The listing builds one solid part. Answer for the finished solid, in the listing's coordinates (mm). A direction names the side the tool comes from. Give positions to 0.01 mm unless a question says otherwise; leave off trailing zeros. Order: outer loops, then holes, each group sorted by start corner. A loop starts at its lowest first (then second) coordinate and runs counter-clockwise, first axis right, second up. Notation, with made-up numbers: (86, 67.25) - (136, 67.25) arc R11 ccw to (136, 79.25) - close; hole circle Ø7 at (4, 67). An arc over 180 degrees is marked (long way). Use a Markdown table: item, result. Add a question column.
1) Flat-ended cylindrical pins translate along their axes: pin 1 (2.5 mm diameter, centred on x = 62, y = 129, fed in from -Z); pin 2 (4 mm diameter, centred on x = 17, y = 22, fed in from +Z); pin 3 (5 mm diameter, centred on x = 61, y = 9, fed in from +Z); pin 4 (2 mm diameter, centred on x = 61, y = 9, fed in from +Z). Find the tip coordinate at first contact, or state that the pin passes through.
2) Find section C-C, the plane y = 83.5. Determine the outline of the cut face in (x, z), plus the area to 3 significant figures.
3) The mould has two halves that part along X. Classify faces 4 (the face through (1, 80, 70)), 5 (the face through (0, 67, 35)), 6 (the face through (58.85, 131.373, 33.031)), 7 (the face through (9.521, 131.966, 33.031)): released by +X, released by -X, zero draft, split by the parting line, or undercut.
4) For faces 1 (the face through (57.185, 10.201, 33.031)), 2 (the face through (60, 168, 2)), 3 (the face through (68, 79, 36)), determine the directions among +Z, -Z, +X, -X, +Y, -Y from which every point of the face is accessible in a straight line to the end or side of a thin tool.
5) Find section A-A, the plane z = 52.5. State how many separate pieces and enclosed holes the cut face has, plus the area to 3 significant figures.
6) Straight lines are drawn through the part: line 1 (Y direction, x = 61, z = 67.85); line 2 (Y direction, x = 61, z = 43); line 3 (X direction, y = 128, z = 67.5). For each, find the intervals that lie inside material, in ascending order.
7) Find section B-B, the plane y = 145. Determine the outline of the cut face in (x, z), plus the area to 3 significant figures.
from build123d import *

# Parameters (mm, degrees)
CROQUIS1_W              = 70
CROQUIS1_H              = 160
SALIENTE_EXTRUIR1_DEPTH = 70
VACIADO1_T              = -2
CROQUIS2_W              = 13
CROQUIS2_H              = 19
CORTAR_EXTRUIR1_DEPTH   = 188.413980268
CORTAR_EXTRUIR2_DEPTH   = 188.413980268
CORTAR_EXTRUIR3_DEPTH   = 188.413980268
CROQUIS5_R              = 5
CROQUIS5_R_2            = 3
SALIENTE_EXTRUIR2_DEPTH = 67
CROQUIS6_R              = 3.05
CROQUIS6_R_2            = 1.4
SALIENTE_EXTRUIR3_DEPTH = 2
SALIENTE_EXTRUIR4_DEPTH = 4
CROQUIS8_R              = 4
CORTAR_EXTRUIR4_DEPTH   = 67


with BuildPart() as part:
    # Croquis1 → Saliente-Extruir1 (new body)
    with BuildSketch(Plane.XY):
        with Locations((35, 80)):
            Rectangle(CROQUIS1_W, CROQUIS1_H)
    extrude(amount=SALIENTE_EXTRUIR1_DEPTH)

    # Vaciado1
    vaciado1_openings = [part.faces().sort_by_distance(p)[0] for p in [
        (35, 80, 70),
    ]]
    offset(amount=VACIADO1_T, openings=vaciado1_openings, kind=Kind.INTERSECTION)

    # Croquis2 → Cortar-Extruir1 (cut, through all)
    with BuildSketch(Plane.XY.offset(2)):
        with Locations((60, 147)):
            Rectangle(CROQUIS2_W, CROQUIS2_H)
    extrude(amount=-CORTAR_EXTRUIR1_DEPTH, mode=Mode.SUBTRACT)

    # Croquis3 → Cortar-Extruir2 (cut, through all)
    with BuildSketch(Plane.XY.offset(2)):
        with BuildLine():
            Line((29.75, 14.573472877), (40.25, 14.573472877))
            ThreePointArc((40.25, 14.573472877), (44, 10.823472877), (40.25, 7.073472877))
            Line((40.25, 7.073472877), (29.75, 7.073472877))
            ThreePointArc((29.75, 7.073472877), (26, 10.823472877), (29.75, 14.573472877))
        make_face()
    extrude(amount=-CORTAR_EXTRUIR2_DEPTH, mode=Mode.SUBTRACT)

    # Croquis4 → Cortar-Extruir3 (cut, through all)
    with BuildSketch(Plane(origin=(2, 0, 0), x_dir=(0, 0, -1), z_dir=(1, 0, 0))):
        with BuildLine():
            Line((-28, 148), (-20, 148))
            ThreePointArc((-20, 148), (-17, 145), (-20, 142))
            Line((-20, 142), (-28, 142))
            ThreePointArc((-28, 142), (-31, 145), (-28, 148))
        make_face()
    extrude(amount=-CORTAR_EXTRUIR3_DEPTH, mode=Mode.SUBTRACT)

    # Croquis5 → Saliente-Extruir2 (add)
    # profile 1 of 4: a face of its own
    with BuildSketch(Plane.XY.offset(2)):
        with Locations(Location((9, 128, 0), (0, 0, 180))):
            Circle(CROQUIS5_R)
        with Locations((9, 128)):
            Circle(CROQUIS5_R_2, mode=Mode.SUBTRACT)
    # profile 2 of 4: a face of its own
    with BuildSketch(Plane.XY.offset(2)):
        with Locations(Location((9, 9, 0), (0, 0, 180))):
            Circle(CROQUIS5_R)
        with Locations((9, 9)):
            Circle(CROQUIS5_R_2, mode=Mode.SUBTRACT)
    # profile 3 of 4: a face of its own
    with BuildSketch(Plane.XY.offset(2)):
        with Locations(Location((61, 128, 0), (0, 0, 180))):
            Circle(CROQUIS5_R)
        with Locations((61, 128)):
            Circle(CROQUIS5_R_2, mode=Mode.SUBTRACT)
    # profile 4 of 4: a face of its own
    with BuildSketch(Plane.XY.offset(2)):
        with Locations(Location((61, 9, 0), (0, 0, 180))):
            Circle(CROQUIS5_R)
        with Locations((61, 9)):
            Circle(CROQUIS5_R_2, mode=Mode.SUBTRACT)
    extrude(amount=SALIENTE_EXTRUIR2_DEPTH)

    # Croquis6 → Saliente-Extruir3 (add)
    # profile 1 of 4: a face of its own
    with BuildSketch(Plane.XY.offset(69)):
        with Locations((9, 128)):
            Circle(CROQUIS6_R)
        with Locations((9, 128)):
            Circle(CROQUIS6_R_2, mode=Mode.SUBTRACT)
    # profile 2 of 4: a face of its own
    with BuildSketch(Plane.XY.offset(69)):
        with Locations((61, 128)):
            Circle(CROQUIS6_R)
        with Locations((61, 128)):
            Circle(CROQUIS6_R_2, mode=Mode.SUBTRACT)
    # profile 3 of 4: a face of its own
    with BuildSketch(Plane.XY.offset(69)):
        with Locations((61, 9)):
            Circle(CROQUIS6_R)
        with Locations((61, 9)):
            Circle(CROQUIS6_R_2, mode=Mode.SUBTRACT)
    # profile 4 of 4: a face of its own
    with BuildSketch(Plane.XY.offset(69)):
        with Locations((9, 9)):
            Circle(CROQUIS6_R)
        with Locations((9, 9)):
            Circle(CROQUIS6_R_2, mode=Mode.SUBTRACT)
    extrude(amount=-SALIENTE_EXTRUIR3_DEPTH)

    # Croquis7 → Saliente-Extruir4 (add)
    # profile 1 of 2: a face of its own
    with BuildSketch(Plane(origin=(0, 0, 0), x_dir=(-1, 0, 0), z_dir=(0, 0, -1))):
        with BuildLine():
            Line((-70, 160), (-60, 160))
            Line((-60, 160), (-60, 176))
            ThreePointArc((-60, 176), (-61.171572875, 178.828427125), (-64, 180))
            Line((-64, 180), (-66, 180))
            ThreePointArc((-66, 180), (-68.828427125, 178.828427125), (-70, 176))
            Line((-70, 176), (-70, 160))
        make_face()
        with BuildLine():
            Line((-66, 177.5), (-64, 177.5))
            ThreePointArc((-64, 177.5), (-62.5, 176), (-64, 174.5))
            Line((-64, 174.5), (-66, 174.5))
            ThreePointArc((-66, 174.5), (-67.5, 176), (-66, 177.5))
        make_face(mode=Mode.SUBTRACT)
    # profile 2 of 2: a face of its own
    with BuildSketch(Plane(origin=(0, 0, 0), x_dir=(-1, 0, 0), z_dir=(0, 0, -1))):
        with BuildLine():
            Line((0, 160), (-10, 160))
            Line((-10, 160), (-10, 176))
            ThreePointArc((-10, 176), (-8.828427125, 178.828427125), (-6, 180))
            Line((-6, 180), (-4, 180))
            ThreePointArc((-4, 180), (-1.171572875, 178.828427125), (0, 176))
            Line((0, 176), (0, 160))
        make_face()
        with BuildLine():
            Line((-6, 177.5), (-4, 177.5))
            ThreePointArc((-4, 177.5), (-2.5, 176), (-4, 174.5))
            Line((-4, 174.5), (-6, 174.5))
            ThreePointArc((-6, 174.5), (-7.5, 176), (-6, 177.5))
        make_face(mode=Mode.SUBTRACT)
    extrude(amount=-SALIENTE_EXTRUIR4_DEPTH)

    # Croquis8 → Cortar-Extruir4 (cut)
    with BuildSketch(Plane(origin=(0, 0, 0), x_dir=(-1, 0, 0), z_dir=(0, 0, -1))):
        with Locations((-61, 128)):
            Circle(CROQUIS8_R)
        with Locations((-9, 128)):
            Circle(CROQUIS8_R)
        with Locations((-61, 9)):
            Circle(CROQUIS8_R)
        with Locations((-9, 9)):
            Circle(CROQUIS8_R)
    extrude(amount=-CORTAR_EXTRUIR4_DEPTH, mode=Mode.SUBTRACT)


solid = part.part
The answers:
| question | item | result |
|---|---|---|
| 1 | pin 1 | z = 67 |
| 1 | pin 2 | z = 2 |
| 1 | pin 3 | z = 69 |
| 1 | pin 4 | through |
| 2 | outline | (0, 0) - (70, 0) - (70, 70) - (68, 70) - (68, 2) - (2, 2) - (2, 70) - (0, 70) - close |
| 2 | area | 412 mm2 |
| 3 | face 4 | zero draft |
| 3 | face 5 | released by -X |
| 3 | face 6 | undercut |
| 3 | face 7 | undercut |
| 4 | face 1 | -Z |
| 4 | face 2 | +Z, -Z, +Y |
| 4 | face 3 | +Z |
| 5 | separate pieces | 5 |
| 5 | enclosed holes | 5 |
| 5 | area | 1,020 mm2 |
| 6 | line 1 | 0 to 2, 4 to 7.6, 10.4 to 14, 123 to 126.6, 129.4 to 133, 158 to 160 |
| 6 | line 2 | 0 to 2, 4 to 5, 13 to 14, 123 to 124, 132 to 133, 158 to 160 |
| 6 | line 3 | 0 to 2, 4 to 7.6, 10.4 to 14, 56 to 59.6, 62.4 to 66, 68 to 70 |
| 7 | outline | (0, 0) - (53.5, 0) - (53.5, 2) - (2, 2) - (2, 17) - (0, 17) - close; (0, 31) - (2, 31) - (2, 70) - (0, 70) - close; (66.5, 0) - (70, 0) - (70, 70) - (68, 70) - (68, 2) - (66.5, 2) - close |
| 7 | area | 358 mm2 |
